The model under review builds one solid part; all positions refer to its coordinate system, in mm. Give positions to 0.01 mm unless a question says otherwise; leave off trailing zeros. Order: outer loops, then holes, each group sorted by start corner. A loop starts at its lowest first (then second) coordinate and runs counter-clockwise, first axis right, second up. Notation, with made-up numbers: (51, 76.5) - (79, 76.5) arc R30 ccw to (79, 103.5) - close; hole circle Ø1 at (86, 60). An arc over 180 degrees is marked (long way). Use CSV: the item, a comma, the result in double quotes.
```python
from build123d import *

# Parameters (mm, degrees)
SKETCH1_R           = 1.5
BOSS_EXTRUDE1_DEPTH = 2
SKETCH2_W           = 23
SKETCH2_H           = 12.5
CUT_EXTRUDE1_DEPTH  = 3


with BuildPart() as part:
    # Sketch1 → Boss-Extrude1 (new body)
    with BuildSketch(Plane(origin=(0, 0, 0), x_dir=(1, 0, 0), z_dir=(0, 1, 0))):
        with BuildLine():
            Line((-9.12, -3.457764929), (-9.12, -8.25))
            Line((-9.12, -8.25), (16.63, -8.25))
            Line((16.63, -8.25), (16.63, -20))
            ThreePointArc((16.63, -20), (20.13, -23.5), (23.63, -20))
            Line((23.63, -20), (23.63, 20))
            ThreePointArc((23.63, 20), (20.13, 23.5), (16.63, 20))
            Line((16.63, 20), (16.63, 8.25))
            Line((16.63, 8.25), (-9.12, 8.25))
            Line((-9.12, 8.25), (-9.12, 3.5))
            Line((-9.12, 3.5), (-10.99, 3.5))
            ThreePointArc((-10.99, 3.5), (-14.49, 0), (-10.99, -3.5))
            Line((-10.99, -3.5), (-9.12, -3.457764929))
        make_face()
        with Locations((-10.99, 0)):
            Circle(SKETCH1_R, mode=Mode.SUBTRACT)
        with Locations((20.01, 0)):
            Circle(SKETCH1_R, mode=Mode.SUBTRACT)
        with Locations((20.13, 20)):
            Circle(SKETCH1_R, mode=Mode.SUBTRACT)
        with Locations((20.13, -20)):
            Circle(SKETCH1_R, mode=Mode.SUBTRACT)
    extrude(amount=BOSS_EXTRUDE1_DEPTH)

    # Sketch2 → Cut-Extrude1 (cut, through all)
    with BuildSketch(Plane(origin=(0, 2, 0), x_dir=(1, 0, 0), z_dir=(0, 1, 0))):
        with Locations((4.51, 0)):
            Rectangle(SKETCH2_W, SKETCH2_H)
    extrude(amount=-CUT_EXTRUDE1_DEPTH, mode=Mode.SUBTRACT)


solid = part.part
```
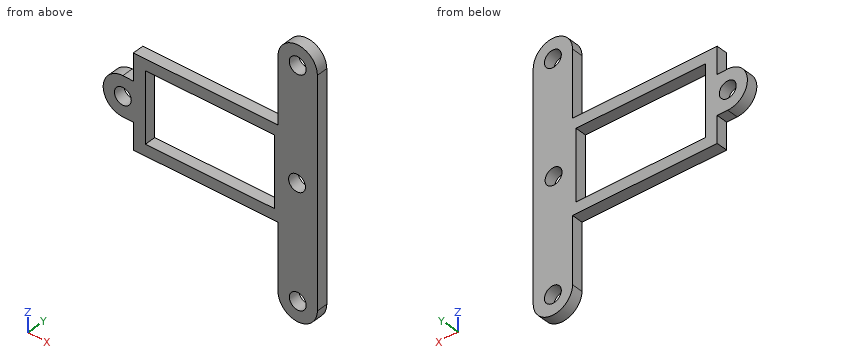
Item 1: Take a section at B-B, the plane x = 4.5. Give the boundary of the cut face in (y, z).
Results list:
outline,"(0, -8.25) - (2, -8.25) - (2, -6.25) - (0, -6.25) - close; (0, 6.25) - (2, 6.25) - (2, 8.25) - (0, 8.25) - close"
Item 2: Wall thickness on L1, parallel to Z at x = 20.13, y = 1.2; L2, parallel to Z at x = 0, y = 1; L3, parallel to X at y = 0.7, z = -20: over which ranges is each line inside the solid? List them lowest first.
Results list:
L1,"z = -23.5 to -21.5, -18.5 to -1.5, 1.5 to 18.5, 21.5 to 23.5"
L2,"z = -8.25 to -6.25, 6.25 to 8.25"
L3,"x = 16.63 to 18.63, 21.63 to 23.63"
Item 3: Take a section at C-C, the plane y = 0.35. Give the boundary of the cut face in (x, z), and give its area (3 significant figures).
Results list:
outline,"(-10.99, -3.5) - (-9.12, -3.5) - (-9.12, -8.25) - (16.63, -8.25) - (16.63, -20) arc R3.5 ccw to (23.63, -20) - (23.63, 20) arc R3.5 ccw to (16.63, 20) - (16.63, 8.25) - (-9.12, 8.25) - (-9.12, 3.46) - (-10.99, 3.5) arc R3.5 ccw to start; hole circle Ø3 at (-10.99, 0); hole (-6.99, -6.25) - (16.01, -6.25) - (16.01, 6.25) - (-6.99, 6.25) - close; hole circle Ø3 at (20.01, 0); hole circle Ø3 at (20.13, -20); hole circle Ø3 at (20.13, 20)"
area,"460 mm2"
Item 4: Take a section at D-D, the plane x = 20.13. Give the boundary of the cut face in (y, z).
Results list:
outline,"(0, -23.5) - (2, -23.5) - (2, -21.5) - (0, -21.5) - close; (0, -18.5) - (2, -18.5) - (2, -1.5) - (0, -1.5) - close; (0, 1.5) - (2, 1.5) - (2, 18.5) - (0, 18.5) - close; (0, 21.5) - (2, 21.5) - (2, 23.5) - (0, 23.5) - close"
Item 5: Clearance check with flat-ended pins moving along their axes: pin 1 (1 mm diameter, centred on x = 0.5, y = 1.5, fed in from +Z); pin 2 (1 mm diameter, centred on y = 1.5, z = 16.5, fed in from -X). State where each tip first meets the part, or that it passes through.
Results list:
pin 1,"stops at z = 8.25"
pin 2,"stops at x = 16.63"
Item 6: Take a section at A-A, the plane z = 0. Give the boundary of the cut face in (x, y).
Results list:
outline,"(-14.49, 0) - (-12.49, 0) - (-12.49, 2) - (-14.49, 2) - close; (-9.49, 0) - (-6.99, 0) - (-6.99, 2) - (-9.49, 2) - close; (16.01, 0) - (18.51, 0) - (18.51, 2) - (16.01, 2) - close; (21.51, 0) - (23.63, 0) - (23.63, 2) - (21.51, 2) - close"
